Input: part model. Units: mm. Frame: model coordinates. A direction names the side the tool comes from. Round coordinates to 2 decimals unless told otherwise and drop trailing zeros. Write each loop counter-clockwise with the first axis right and the second up, starting at its lowest first coordinate (ties: lowest second). Pieces come first, ordered by that corner, then holes. Notation, with made-up numbers: (86.25, 69.5) -> (138.25, 69.5) arc R13 ccw to (138.25, 91.5) -> close; hole circle Ø10 at (-8.75, -10.5). An arc over 180 degrees is marked (long way). Write item = value, one per line.
```python
from build123d import *

# Parameters (mm, degrees)
SKETCH1_R           = 13
BOSS_EXTRUDE1_DEPTH = 20
SKETCH2_R           = 10.1
CUT_EXTRUDE1_DEPTH  = 4.5
SKETCH3_R           = 4.25
CUT_EXTRUDE2_DEPTH  = 2.6
SKETCH4_R           = 2.125
CUT_EXTRUDE3_DEPTH  = 10
SKETCH5_R           = 2
CUT_EXTRUDE4_DEPTH  = 13.5
SKETCH6_R           = 1.1
CUT_EXTRUDE5_DEPTH  = 28.166155414
SKETCH7_R           = 2
CUT_EXTRUDE6_DEPTH  = 6


with BuildPart() as part:
    # Sketch1 → Boss-Extrude1 (new body)
    with BuildSketch(Plane.XY):
        Circle(SKETCH1_R)
    extrude(amount=BOSS_EXTRUDE1_DEPTH)

    # Sketch2 → Cut-Extrude1 (cut)
    with BuildSketch(Plane.XY.offset(20)):
        Circle(SKETCH2_R)
    extrude(amount=-CUT_EXTRUDE1_DEPTH, mode=Mode.SUBTRACT)

    # Sketch3 → Cut-Extrude2 (cut)
    with BuildSketch(Plane.XY.offset(15.5)):
        Circle(SKETCH3_R)
    extrude(amount=-CUT_EXTRUDE2_DEPTH, mode=Mode.SUBTRACT)

    # Sketch4 → Cut-Extrude3 (cut)
    with BuildSketch(Plane(origin=(0, 0, 0), x_dir=(-1, 0, 0), z_dir=(0, 0, -1))):
        Circle(SKETCH4_R)
    extrude(amount=-CUT_EXTRUDE3_DEPTH, mode=Mode.SUBTRACT)

    # Sketch5 → Cut-Extrude4 (cut)
    with BuildSketch(Plane(origin=(0, 0, 0), x_dir=(-1, 0, 0), z_dir=(0, 0, -1))):
        with Locations((0, 7)):
            Circle(SKETCH5_R)
        with Locations((7, 0)):
            Circle(SKETCH5_R)
        with Locations((0, -7)):
            Circle(SKETCH5_R)
    extrude(amount=-CUT_EXTRUDE4_DEPTH, mode=Mode.SUBTRACT)

    # Sketch6 → Cut-Extrude5 (cut, through all)
    with BuildSketch(Plane(origin=(0, 0, 0), x_dir=(-1, 0, 0), z_dir=(0, 0, -1))):
        with Locations(Location((0, 7, 0), (0, 0, 180))):
            Circle(SKETCH6_R)
        with Locations(Location((7, 0, 0), (0, 0, 180))):
            Circle(SKETCH6_R)
        with Locations(Location((0, -7, 0), (0, 0, 180))):
            Circle(SKETCH6_R)
    extrude(amount=-CUT_EXTRUDE5_DEPTH, mode=Mode.SUBTRACT)

    # Sketch7 → Cut-Extrude6 (cut)
    with BuildSketch(Plane(origin=(0, 0, 0), x_dir=(-1, 0, 0), z_dir=(0, 0, -1))):
        with Locations((-6, 5)):
            Circle(SKETCH7_R)
        with Locations(Location((-6, -5, 0), (0, 0, 180))):
            Circle(SKETCH7_R)
    extrude(amount=-CUT_EXTRUDE6_DEPTH, mode=Mode.SUBTRACT)


solid = part.part
```
1) Cut plane B-B (x = -7). Return the cut outline in (y, z), and give its area (3 significant figures).
Solutions:
outline = (-10.95, 0) -> (-2, 0) -> (-2, 13.5) -> (-1.1, 13.5) -> (-1.1, 15.5) -> (-7.28, 15.5) -> (-7.28, 20) -> (-10.95, 20) -> close; (1.1, 13.5) -> (2, 13.5) -> (2, 0) -> (10.95, 0) -> (10.95, 20) -> (7.28, 20) -> (7.28, 15.5) -> (1.1, 15.5) -> close
area = 314 mm^2
2) Cut plane D-D (z = 8). Return the cut outline in (x, y) (3 decimals).
Solutions:
outline = circle Ø26 at (0, 0); hole circle Ø4 at (-7, 0); hole circle Ø4.25 at (0, 0); hole circle Ø4 at (0, -7); hole circle Ø4 at (0, 7)
3) Access query for faces 4 (the face through (-1, 6, 13.5)), 5 (the face through (-5.984, 0.421, 14.486)), 6 (the face through (0, 0, 12.9)). Directions: +Z, -Z, +X, -X, +Y, -Y. A direction counts if a zero-diameter tool reaches every point of the face in a straight line with its end or side. Return the directions, or none.
Solutions:
face_4 = -Z
face_5 = +Z, -Z
face_6 = +Z
4) First-contact query: P1, Ø3, axis at x = -3, z = 7.5, coming from the +Y side; P2, Ø12, axis at x = 4.5, z = 11, coming from the -Y side; P3, Ø4, axis at x = -1.5, y = -1.5, coming from the +Z side; P4, Ø8, axis at x = 7, z = 10.5, coming from the +Y side. Flat tips, straight axial feed; report the tip coordinate or a pass-through.
Solutions:
P1 = 12.91
P2 = -13
P3 = 12.9
P4 = 12.65
5) Line query: L1, parallel to Y at x = 0, z = 2.75 (3 decimals); L2, parallel to Y at x = 6.25, z = 5; L3, parallel to Z at x = -1.25, y = -4.5. Output: solid intervals per line, ascending. Write a range as from..to.
Solutions:
L1 = -13..-9, -5..-2.125, 2.125..5, 9..13
L2 = -11.4..-6.98, -3.02..3.02, 6.98..11.4
L3 = 0..15.5
6) Cut plane C-C (z = 3.5). Return the cut outline in (x, y) (3 decimals), and give its area (3 significant figures).
Solutions:
outline = circle Ø26 at (0, 0); hole circle Ø4 at (-7, 0); hole circle Ø4.25 at (0, 0); hole circle Ø4 at (0, -7); hole circle Ø4 at (0, 7); hole circle Ø4 at (6, -5); hole circle Ø4 at (6, 5)
area = 454 mm^2
7) Cut plane A-A (y = 0). Return the cut outline in (x, z) (3 decimals), and give its area (3 significant figures).
Solutions:
outline = (-13, 0) -> (-9, 0) -> (-9, 13.5) -> (-8.1, 13.5) -> (-8.1, 15.5) -> (-10.1, 15.5) -> (-10.1, 20) -> (-13, 20) -> close; (-5.9, 13.5) -> (-5, 13.5) -> (-5, 0) -> (-2.125, 0) -> (-2.125, 10) -> (2.125, 10) -> (2.125, 0) -> (13, 0) -> (13, 20) -> (10.1, 20) -> (10.1, 15.5) -> (4.25, 15.5) -> (4.25, 12.9) -> (-4.25, 12.9) -> (-4.25, 15.5) -> (-5.9, 15.5) -> close
area = 306 mm^2
8) Draft query along X for faces 1 (the face through (-10.316, -7.91, 9.86)), 2 (the face through (0, -3, 0)), 3 (the face through (-1.142, 1.792, 4.93)). Return one class per face: +X half, -X half, draft (parallel to the pull), parting line (faces both ways), or undercut.
Solutions:
face_1 = parting line
face_2 = draft
face_3 = undercut
